Source: CAD feature listing. Evaluate the final solid. Frame: model axes, mm. Face numbers are marked on the shaded views. A direction names the side the tool comes from. Give positions to 0.01 mm unless a question says otherwise; leave off trailing zeros. Order: outer loops, then holes, each group sorted by start corner. A loop starts at its lowest first (then second) coordinate and runs counter-clockwise, first axis right, second up.
1) Section C-C, the plane x = 42. Return loops of the section in (y, z), plus the area to 3 significant figures.
2) Section A-A, the plane z = 4.5. Return loops of the section in (x, y).
3) Access query for the marked faces 4, 5, 6 and 7. Directions: +Z, -Z, +X, -X, +Y, -Y. A direction counts if a zero-diameter tool reaches every point of the face in a straight line with its end or side. Return the directions, or none.
4) First-contact query: P1, Ø10, axis at y = -10.5, z = 27, coming from the -X side; P2, Ø6.5, axis at x = 47.5, y = -23, coming from the +Z side; P3, Ø6, axis at y = -21.5, z = 25, coming from the +X side. Flat tips, straight axial feed; report the tip coordinate or a pass-through.
5) Material intervals for line 1 (X direction, y = -19, z = 2); line 2 (Z direction, x = 14, y = -26.5); line 3 (X direction, y = -8.5, z = 30.5), sorted ascending.
6) Draft query along X for the marked faces 1, 2 and 3. Return one class per face: released by +X, released by -X, zero draft, split by the parting line, or undercut.
7) Section B-B, the plane y = -24. Return loops of the section in (x, z), plus the area to 3 significant figures.
8) Section D-D, the plane z = 30. Return loops of the section in (x, y), plus the area to 3 significant figures.
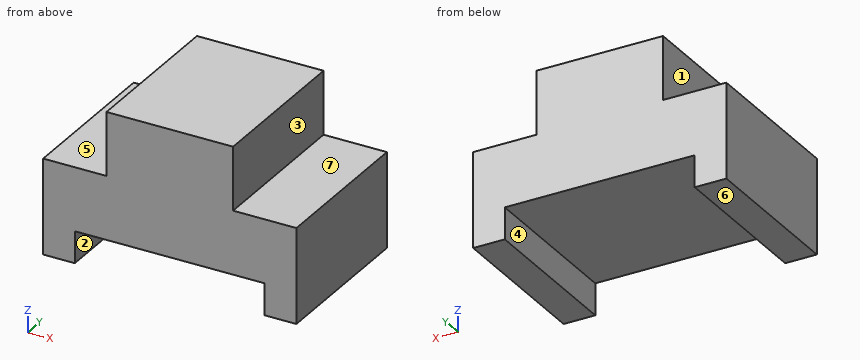
```python
from build123d import *

# Parameters (mm, degrees)
F0_W     = 50.8
F0_H     = 31.75
F1_DEPTH = 31.75
F2_W     = 12.7
F2_H     = 12.7
F2_W_2   = 38.1
F2_H_2   = 6.35
F3_DEPTH = 56.642


with BuildPart() as f1:
    # F0 (on Top) → F1 (new body)
    with BuildSketch(Plane.XY):
        with Locations((25.4, -15.875)):
            Rectangle(F0_W, F0_H)
    extrude(amount=F1_DEPTH)

    # F2 (on Front) → F3 (cut)
    with BuildSketch(Plane.XZ):
        with Locations((6.35, 25.4)):
            Rectangle(F2_W, F2_H)
        with Locations((44.45, 25.4)):
            Rectangle(F2_W, F2_H)
        with Locations((25.4, 3.175)):
            Rectangle(F2_W_2, F2_H_2)
    extrude(amount=F3_DEPTH, mode=Mode.SUBTRACT)


solid = f1.part
```
From the geometry:
1. outline: (-31.75, 6.35) - (0, 6.35) - (0, 19.05) - (-31.75, 19.05) - close
1. area: 403 mm2
2. outline: (0, -31.75) - (6.35, -31.75) - (6.35, 0) - (0, 0) - close; (44.45, -31.75) - (50.8, -31.75) - (50.8, 0) - (44.45, 0) - close
3. face 4: -Z, +Y, -Y
3. face 5: +Z, -X, +Y, -Y
3. face 6: -Z, +X, -X, +Y, -Y
3. face 7: +Z, +X, +Y, -Y
4. P1: stops at x = 12.7
4. P2: stops at z = 19.05
4. P3: stops at x = 38.1
5. line 1: x = 0 to 6.35, 44.45 to 50.8
5. line 2: z = 6.35 to 31.75
5. line 3: x = 12.7 to 38.1
6. face 1: released by -X
6. face 2: undercut
6. face 3: released by +X
7. outline: (0, 0) - (6.35, 0) - (6.35, 6.35) - (44.45, 6.35) - (44.45, 0) - (50.8, 0) - (50.8, 19.05) - (38.1, 19.05) - (38.1, 31.75) - (12.7, 31.75) - (12.7, 19.05) - (0, 19.05) - close
7. area: 1,050 mm2
8. outline: (12.7, -31.75) - (38.1, -31.75) - (38.1, 0) - (12.7, 0) - close
8. area: 806 mm2
